Build history of the part. All positions in model axes, mm. Face numbers are marked on the shaded views. A direction names the side the tool comes from. Round coordinates to 2 decimals unless told otherwise and drop trailing zeros. Write each loop counter-clockwise with the first axis right and the second up, starting at its lowest first coordinate (ties: lowest second). Pieces come first, ordered by that corner, then holes. Notation, with made-up numbers: (41.25, 35.5) -> (57.25, 35.5) arc R24 ccw to (57.25, 51.5) -> close; hole circle Ø5 at (64.25, 25.25). An arc over 180 degrees is marked (long way). Answer as CSV lines item,"result".
from build123d import *

# Parameters (mm, degrees)
BOSS_EXTRUDE2_DEPTH      = 22.5
BOSS_EXTRUDE2_DEPTH_BACK = 22.5
SKETCH7_W                = 41
SKETCH7_H                = 45
CUT_EXTRUDE4_DEPTH       = 41.5
CUT_EXTRUDE4_DEPTH_BACK  = 22.5
SKETCH8_R                = 1.25
CUT_EXTRUDE5_DEPTH       = 18.5
SKETCH9_R                = 1.25
CUT_EXTRUDE6_DEPTH       = 58.5
SKETCH10_R               = 3.181768177
CUT_EXTRUDE7_DEPTH       = 1


with BuildPart() as part:
    # Sketch6 → Boss-Extrude2 (new body, two sides)
    with BuildSketch(Plane(origin=(0, 0, 0), x_dir=(0, 0, -1), z_dir=(1, 0, 0))) as boss_extrude2_sk:
        with BuildLine():
            Line((-22.5, 0), (-22.5, 43.5))
            Line((-22.5, 43.5), (22.5, 43.5))
            Line((22.5, 43.5), (22.5, 0))
            ThreePointArc((22.5, 0), (0, -22.5), (-22.5, 0))
        make_face()
    extrude(amount=BOSS_EXTRUDE2_DEPTH)
    extrude(boss_extrude2_sk.sketch, amount=-BOSS_EXTRUDE2_DEPTH_BACK)

    # Sketch7 → Cut-Extrude4 (cut, two sides)
    with BuildSketch(Plane(origin=(0, 0, 0), x_dir=(1, 0, 0), z_dir=(0, 1, 0))) as cut_extrude4_sk:
        Rectangle(SKETCH7_W, SKETCH7_H)
    extrude(amount=CUT_EXTRUDE4_DEPTH, mode=Mode.SUBTRACT)
    extrude(cut_extrude4_sk.sketch, amount=-CUT_EXTRUDE4_DEPTH_BACK, mode=Mode.SUBTRACT)

    # Sketch8 → Cut-Extrude5 (cut)
    with BuildSketch(Plane(origin=(0, 43.5, 0), x_dir=(1, 0, 0), z_dir=(0, 1, 0))):
        with Locations((-5, 5)):
            Circle(SKETCH8_R)
        with Locations((5, -5)):
            Circle(SKETCH8_R)
        with Locations((5, 5)):
            Circle(SKETCH8_R)
        with Locations((-5, -5)):
            Circle(SKETCH8_R)
    extrude(amount=-CUT_EXTRUDE5_DEPTH, mode=Mode.SUBTRACT)

    # Sketch9 → Cut-Extrude6 (cut)
    with BuildSketch(Plane.ZY.offset(22.5)):
        with Locations((0, 7)):
            Circle(SKETCH9_R)
        with Locations((0, -7)):
            Circle(SKETCH9_R)
        with Locations((-7, 0)):
            Circle(SKETCH9_R)
        with Locations((7, 0)):
            Circle(SKETCH9_R)
    extrude(amount=-CUT_EXTRUDE6_DEPTH, mode=Mode.SUBTRACT)

    # Sketch10 → Cut-Extrude7 (cut)
    with BuildSketch(Plane.ZY.offset(22.5)):
        Circle(SKETCH10_R)
    extrude(amount=-CUT_EXTRUDE7_DEPTH, mode=Mode.SUBTRACT)


solid = part.part
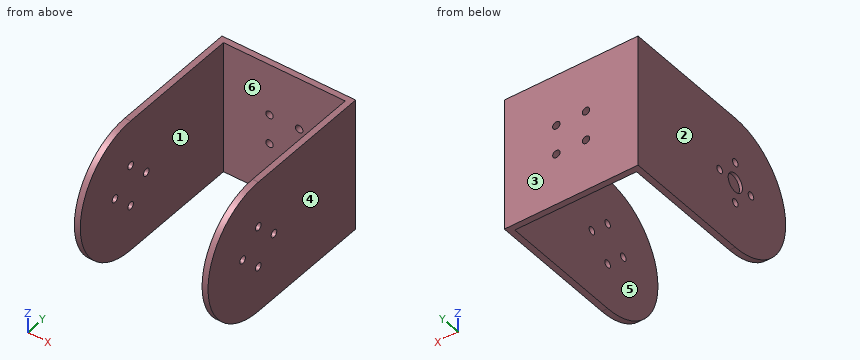
1. Which spindle directions (+Z, -Z, +X, -X, +Y, -Y) get a long thin tool onto all of the face, cutting with end or side? Do the marked faces 1 and 2. Say none if no direction does.
Results found:
face 1,"+Z, -Z, -Y"
face 2,"+Z, -Z, -X, +Y, -Y"
2. Cut at C-C, the plane y = 27. Write the cut outline in (x, z).
Results found:
outline,"(-22.5, -22.5) -> (-20.5, -22.5) -> (-20.5, 22.5) -> (-22.5, 22.5) -> close; (20.5, -22.5) -> (22.5, -22.5) -> (22.5, 22.5) -> (20.5, 22.5) -> close"
3. Probe line 1 along Y through (x, z) = (-21.8, 0); line 2 along X through (y, z) = (42.05, -5); line 3 along Y through (x, z) = (21.2, 0). List the from-to ranges inside material, lowest first.
Results found:
line 1,"y = -22.5 to -8.25, -5.75 to -3.18, 3.18 to 5.75, 8.25 to 43.5"
line 2,"x = -22.5 to -6.25, -3.75 to 3.75, 6.25 to 22.5"
line 3,"y = -22.5 to -8.25, -5.75 to 5.75, 8.25 to 43.5"
4. Drop flat-ended pins along their axis: pin 1 Ø3 at (y, z) = (0.5, 1) entering from -X; pin 2 Ø2 at (x, z) = (5.5, 1) entering from -Y. Give the stop position or say it passes through.
Results found:
pin 1,"stops at x = -21.5"
pin 2,"stops at y = 41.5"
5. Mould opens along X. For the marked faces 3, 4, 5 and 6 say: +X half, -X half, draft (parallel to the pull), parting line (faces both ways), or undercut.
Results found:
face 3,"draft"
face 4,"+X half"
face 5,"undercut"
face 6,"undercut"
6. Cut at D-D, the plane y = 7. Write the cut outline in (x, z), then the cut area to 3 significant figures.
Results found:
outline,"(-22.5, -22.5) -> (-20.5, -22.5) -> (-20.5, -1.25) -> (-22.5, -1.25) -> close; (-22.5, 1.25) -> (-20.5, 1.25) -> (-20.5, 22.5) -> (-22.5, 22.5) -> close; (20.5, -22.5) -> (22.5, -22.5) -> (22.5, -1.25) -> (20.5, -1.25) -> close; (20.5, 1.25) -> (22.5, 1.25) -> (22.5, 22.5) -> (20.5, 22.5) -> close"
area,"170 mm2"
7. Cut at B-B, the plane x = 5. Write the cut outline in (y, z).
Results found:
outline,"(41.5, -22.5) -> (43.5, -22.5) -> (43.5, -6.25) -> (41.5, -6.25) -> close; (41.5, -3.75) -> (43.5, -3.75) -> (43.5, 3.75) -> (41.5, 3.75) -> close; (41.5, 6.25) -> (43.5, 6.25) -> (43.5, 22.5) -> (41.5, 22.5) -> close"
8. Cut at A-A, the plane z = 0. Write the cut outline in (x, y).
Results found:
outline,"(-22.5, -22.5) -> (-20.5, -22.5) -> (-20.5, -8.25) -> (-22.5, -8.25) -> close; (-22.5, -5.75) -> (-20.5, -5.75) -> (-20.5, 5.75) -> (-22.5, 5.75) -> (-22.5, 3.18) -> (-21.5, 3.18) -> (-21.5, -3.18) -> (-22.5, -3.18) -> close; (-22.5, 8.25) -> (-20.5, 8.25) -> (-20.5, 41.5) -> (20.5, 41.5) -> (20.5, 8.25) -> (22.5, 8.25) -> (22.5, 43.5) -> (-22.5, 43.5) -> close; (20.5, -22.5) -> (22.5, -22.5) -> (22.5, -8.25) -> (20.5, -8.25) -> close; (20.5, -5.75) -> (22.5, -5.75) -> (22.5, 5.75) -> (20.5, 5.75) -> close"
